```python
from build123d import *

# Parameters (mm, degrees)
SKETCH_2_R          = 7
CUT_EXTRUDE_1_DEPTH = 89.746830997


with BuildPart() as part:
    # Эскиз1 → Повернуть1 (revolve)
    with BuildSketch(Plane.XY, mode=Mode.PRIVATE) as revolve_1_sk:
        with BuildLine():
            Line((-16, 0), (-16, 30))
            Line((-16, 30), (-29.5, 30))
            Line((-29.5, 30), (-29.5, 26))
            Line((-29.5, 26), (-60, 26))
            Line((-60, 26), (-60, 20))
            ThreePointArc((-60, 20), (-59.414213562, 18.585786438), (-58, 18))
            Line((-58, 18), (-26.480170025, 18))
            ThreePointArc((-26.480170025, 18), (-25.290395707, 17.607618447), (-24.567466883, 16.584437071))
            Line((-24.567466883, 16.584437071), (-19.5, 0))
            Line((-19.5, 0), (-16, 0))
        make_face()
    revolve(revolve_1_sk.sketch.rotate(Axis((0, 0, 0), (0, 1, 0)), 270), axis=Axis((0, 0, 0), (0, 1, 0)))

    # Эскиз2 → Вырез-Вытянуть1 (cut, through all)
    with BuildSketch(Plane(origin=(0, 26, 0), x_dir=(1, 0, 0), z_dir=(0, 1, 0))):
        with Locations(Location((-45, 0, 0), (0, 0, 270))):
            Circle(SKETCH_2_R)
        with Locations(Location((0, 45, 0), (0, 0, 270))):
            Circle(SKETCH_2_R)
        with Locations(Location((45, 0, 0), (0, 0, 270))):
            Circle(SKETCH_2_R)
        with Locations(Location((0, -45, 0), (0, 0, 270))):
            Circle(SKETCH_2_R)
    extrude(amount=-CUT_EXTRUDE_1_DEPTH, mode=Mode.SUBTRACT)


solid = part.part
```
Check sheet for the modelled part. Datum: model origin and axes. Units: mm. A direction names the side the tool comes from. Round coordinates to 2 decimals unless told otherwise and drop trailing zeros. Order: outer loops, then holes, each group sorted by start corner. A loop starts at its lowest first (then second) coordinate and runs counter-clockwise, first axis right, second up. Notation, with made-up numbers: (30.25, -11.75) -> (48.25, -11.75) arc R18 ccw to (48.25, 3.25) -> close; hole circle Ø5 at (40, 0.5). An arc over 180 degrees is marked (long way). One line per item, written item: value. Start each with the question number.
Q1. Thickness scan on line 1 (X direction, y = 18.25, z = 5); line 2 (X direction, y = 19.5, z = 0); line 3 (Z direction, x = -0.5, y = 26.5). Record the ranges inside material, lowest first.
Q2. Cross-section at B-B (x = -4). Give the number of separate pieces and of enclosed holes in the cut face, and give its area (3 significant figures).
Q3. Mould release check, pull along Z, two halves, no side actions. Record for faces 3 (the face through (12, 18, -25)), 4 (the face through (15.62, 15.21, 3.47)), 5 (the face through (-8.86, 27.97, -28.14)), 6 (the face through (2.103, 22.056, 51.677)): pulls with the +Z half, pulls with the -Z half, needs draft (parallel to the pull), parting line crosses it, or undercut.
Q4. Cross-section at C-C (y = 7). Record the boundary of the cut face in (x, z), and give its area (3 significant figures).
Q5. Gauge pin test, flat ends, axial feed: pin 1 Ø1.5 at (x, z) = (-32.5, -43) entering from +Y; pin 2 Ø5 at (y, z) = (7, 17.5) entering from +X; pin 3 Ø6 at (x, y) = (-14, 9.5) entering from +Z. Record the tip position at first contact, or that the pin passes through.
Q6. Cross-section at A-A (z = 0). Record the boundary of the cut face in (x, y), and give its area (3 significant figures).
Q7. Set-up check for faces 1 (the face through (-6.1, 2.65, -19.37)), 2 (the face through (-28, 26, 12)): record each of +Z, -Z, +X, -X, +Y, -Y from which the full face is reachable in a straight line by a thin tool's end or side.
Completed:
1. line 1: x = -58.76 to -49.9, -40.1 to -15.2, 15.2 to 40.1, 49.9 to 58.76
1. line 2: x = -59.94 to -52, -38 to -16, 16 to 38, 52 to 59.94
1. line 3: z = -29.5 to -15.99, 15.99 to 29.5
2. separate pieces: 4
2. enclosed holes: 0
2. area: 865 mm²
3. face 3: needs draft
3. face 4: undercut
3. face 5: parting line crosses it
3. face 6: undercut
4. outline: circle Ø43.28 at (0, 0); hole circle Ø32 at (0, 0)
4. area: 667 mm²
5. pin 1: stops at y = 26
5. pin 2: stops at x = 15.82
5. pin 3: stops at z = 19.82
6. outline: (-60, 20) arc R2 ccw to (-58, 18) -> (-52, 18) -> (-52, 26) -> (-60, 26) -> close; (-38, 18) -> (-26.48, 18) arc R2 cw to (-24.57, 16.58) -> (-19.5, 0) -> (-16, 0) -> (-16, 30) -> (-29.5, 30) -> (-29.5, 26) -> (-38, 26) -> close; (16, 0) -> (19.5, 0) -> (24.57, 16.58) arc R2 cw to (26.48, 18) -> (38, 18) -> (38, 26) -> (29.5, 26) -> (29.5, 30) -> (16, 30) -> close; (52, 18) -> (58, 18) arc R2 ccw to (60, 20) -> (60, 26) -> (52, 26) -> close
6. area: 812 mm²
7. face 1: -Y
7. face 2: +Y
